Autodesk Inventor part; units mm, degrees
ref_plane "作業平面1" through (0, 0, -12) normal (0, 0, -1) x (-1, 0, 0)
ref_plane "YZ Plane" through (0, 0, 0) normal (1, 0, 0) x (0, 1, 0)
ref_plane "XZ Plane" through (0, 0, 0) normal (0, 1, 0) x (-1, 0, 0)
sketch "スケッチ1" plane through (0, 0, 0) normal (0, 0, 1) x (1, 0, 0)
  circle A0 centre (0, 0) radius 10
  line L0 (-7.5, 6.6144) -> (7.5, 6.6144) construction
  line L1 (7.5, 6.6144) -> (7.5, -6.6144)
  line L2 (7.5, -6.6144) -> (-7.5, -6.6144) construction
  line L3 (-7.5, -6.6144) -> (-7.5, 6.6144)
  dimension "d0" = 20
  dimension "d1" = 15
extrude "押し出し1" add sketch "スケッチ1" along normal blind 25 contours L1 A0 L3
sketch "スケッチ2" plane through (0, 0, 25) normal (0, 0, 1) x (1, 0, 0)
  circle A0 centre (0, 0) radius 3
  dimension "d4" = 6
extrude "押し出し2" add sketch "スケッチ2" along normal blind 2
sketch "スケッチ3" plane through (0, 0, 0) normal (0, 0, -1) x (-1, 0, 0)
  circle A0 centre (0, 0) radius 5
  dimension "d7" = 10
extrude "押し出し3" add sketch "スケッチ3" along normal blind 2
ref_plane "作業平面1" through (0, 0, -12) normal (0, 0, -1) x (-1, 0, 0)
sketch "スケッチ4" plane through (0, 0, -12) normal (0, 0, -1) x (-1, 0, 0)
  circle A0 centre (0, 0) radius 1
  dimension "d11" = 2
extrude "押し出し4" add sketch "スケッチ4" against normal blind 49
properties part number "Motor_400"
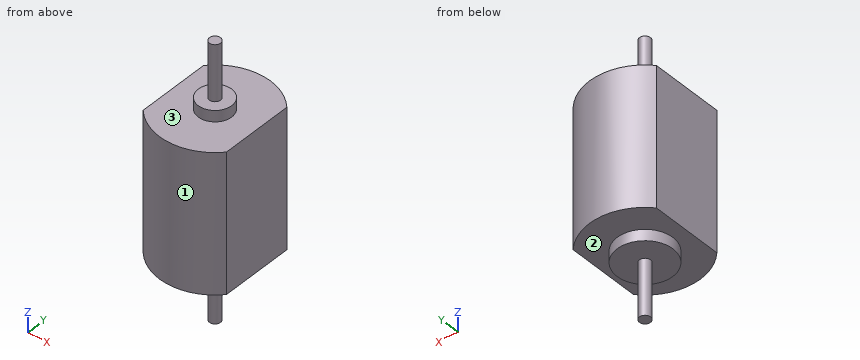
Source: CAD feature listing. Evaluate the final solid. Frame: model axes, mm. Face numbers are marked on the shaded views. A direction names the side the tool comes from. Coordinates: 2 decimals unless noted, no trailing zeros. Write each loop counter-clockwise with the first axis right and the second up, starting at its lowest first coordinate (ties: lowest second). Pieces come first, ordered by that corner, then holes. Notation, with made-up numbers: M 41.5,55.5 L 91.5,55.5 A7 cw 91.5,66.5 Z; hole C -10.5,39 d2. An arc over 180 degrees is marked long. Use a Markdown table: item, result.
1) First-contact query: pin 1 Ø4 at (x, y) = (-5, 7.5) entering from +Z; pin 2 Ø6.5 at (x, y) = (1, -0.5) entering from +Z; pin 3 Ø6 at (x, y) = (0.5, -4) entering from +Z; pin 4 Ø4 at (x, y) = (6, -3) entering from -Z. Flat tips, straight axial feed; report the tip coordinate or a pass-through.
Conclusion:
| item | result |
|---|---|
| pin 1 | stops at z = 25 |
| pin 2 | stops at z = 37 |
| pin 3 | stops at z = 27 |
| pin 4 | stops at z = -2 |
2) Ray query, L1, parallel to Z at x = -2.5, y = 1; L2, parallel to Z at x = -6.25, y = -3.25; L3, parallel to Y at x = -0.25, z = 10. Return the intervals inside material, ascending.
Conclusion:
| item | result |
|---|---|
| L1 | z = -2 to 27 |
| L2 | z = 0 to 25 |
| L3 | y = -10 to 10 |
3) Section A-A, the plane x = 0. Output: boundary loops of the cut face in (y, z), then the cut area to 3 significant figures.
Conclusion:
| item | result |
|---|---|
| outline | M -10,0 L -5,0 L -5,-2 L -1,-2 L -1,-12 L 1,-12 L 1,-2 L 5,-2 L 5,0 L 10,0 L 10,25 L 3,25 L 3,27 L 1,27 L 1,37 L -1,37 L -1,27 L -3,27 L -3,25 L -10,25 Z |
| area | 572 mm^2 |
4) Section D-D, the plane y = 6. Output: boundary loops of the cut face in (x, z), then the cut area to 3 significant figures.
Conclusion:
| item | result |
|---|---|
| outline | M -7.5,0 L 7.5,0 L 7.5,25 L -7.5,25 Z |
| area | 375 mm^2 |
5) Section C-C, the plane z = -4. Output: boundary loops of the cut face in (x, y), then the cut area to 3 significant figures.
Conclusion:
| item | result |
|---|---|
| outline | C 0,0 d2 |
| area | 3.14 mm^2 |
6) Section B-B, the plane y = 0. Output: boundary loops of the cut face in (x, z).
Conclusion:
| item | result |
|---|---|
| outline | M -7.5,0 L -5,0 L -5,-2 L -1,-2 L -1,-12 L 1,-12 L 1,-2 L 5,-2 L 5,0 L 7.5,0 L 7.5,25 L 3,25 L 3,27 L 1,27 L 1,37 L -1,37 L -1,27 L -3,27 L -3,25 L -7.5,25 Z |
7) Reachability of the marked faces 1, 2 and 3 from +Z, -Z, +X, -X, +Y, -Y: full face, straight path, thin tool, end or side. Return the list, or none.
Conclusion:
| item | result |
|---|---|
| face 1 | +Z, -Z, -Y |
| face 2 | -Z |
| face 3 | +Z |
